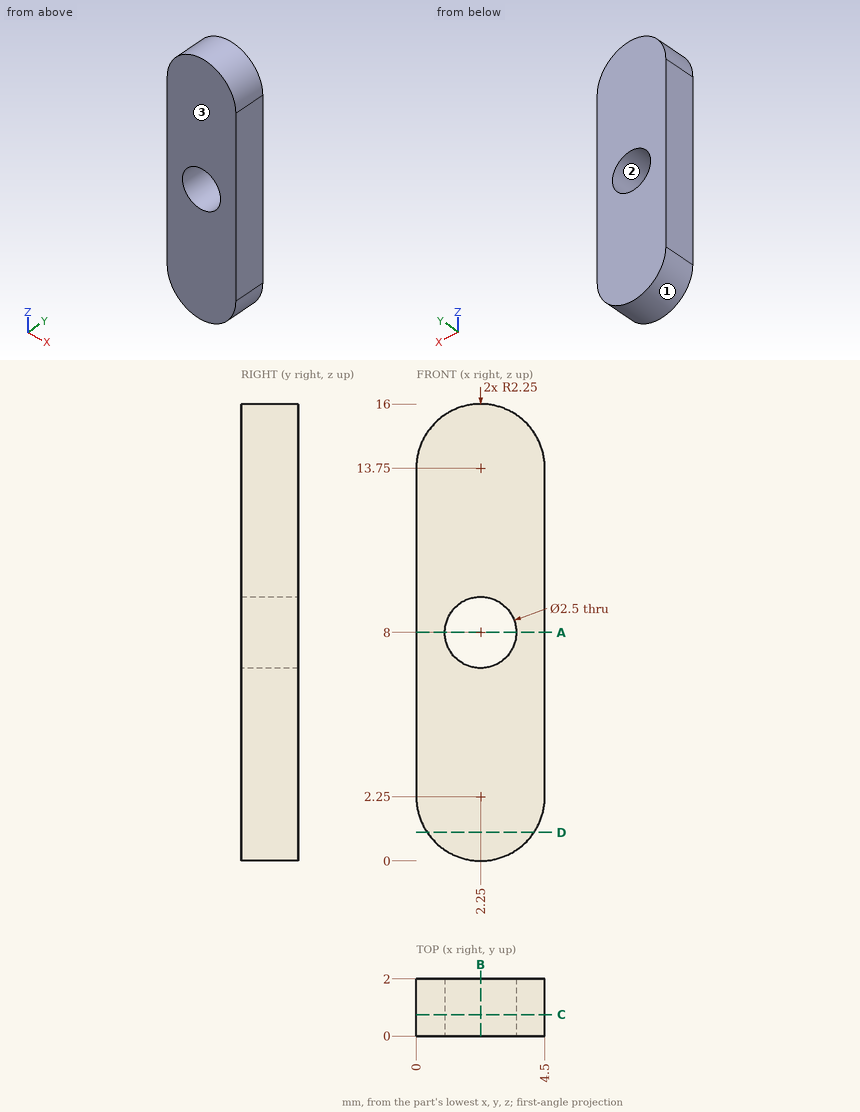
Answer from the drawing. Dimensions are ordinates in mm from the lowest x, y and z of the part. Give positions to 0.01 mm unless a question says otherwise; leave off trailing zeros. Order: outer loops, then holes, each group sorted by start corner. A loop starts at its lowest first (then second) coordinate and runs counter-clockwise, first axis right, second up.
(1) Find section C-C (y = 0.75). Give the vertices of the cut face in (x, z).
(2) Straight lines are drawn through the part: L1, parallel to X at y = 1.2, z = 8; L2, parallel to X at y = 1, z = 9; L3, parallel to Z at x = 2.95, y = 0.85. For each, find the intervals that lie inside material, in ascending order.
(3) Find section A-A (z = 8). Give the vertices of the cut face in (x, y).
(4) Find section D-D (z = 1). Give the vertices of the cut face in (x, y).
(5) Find section B-B (x = 2.25). Give the vertices of the cut face in (y, z).
(6) For a pull along X with two mould halves and no side action, classify the marked faces 1, 2 and 3 as released by +X, released by -X, zero draft, split by the parting line, or undercut.
Result sheet:
1. outline: (0, 2.25) arc R2.25 ccw to (4.5, 2.25) - (4.5, 13.75) arc R2.25 ccw to (0, 13.75) - close; hole circle Ø2.5 at (2.25, 8)
2. L1: x = 0 to 1, 3.5 to 4.5
2. L2: x = 0 to 1.5, 3 to 4.5
2. L3: z = 0.11 to 6.96, 9.04 to 15.89
3. outline: (0, 0) - (1, 0) - (1, 2) - (0, 2) - close; (3.5, 0) - (4.5, 0) - (4.5, 2) - (3.5, 2) - close
4. outline: (0.38, 0) - (4.12, 0) - (4.12, 2) - (0.38, 2) - close
5. outline: (0, 0) - (2, 0) - (2, 6.75) - (0, 6.75) - close; (0, 9.25) - (2, 9.25) - (2, 16) - (0, 16) - close
6. face 1: split by the parting line
6. face 2: undercut
6. face 3: zero draft
